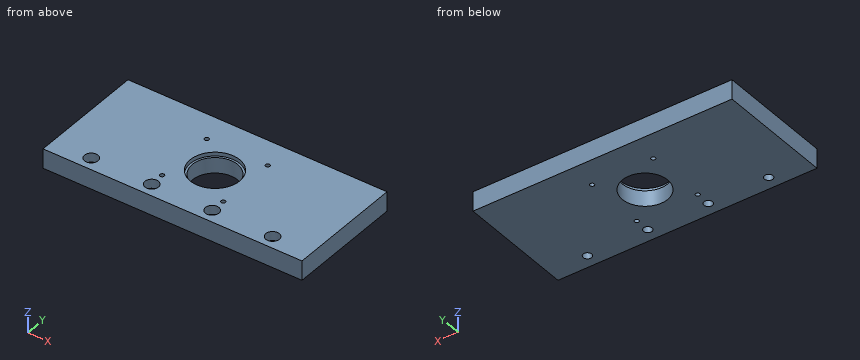
```python
from build123d import *

# Parameters (mm, degrees)
SKETCH_W        = 200
SKETCH_H        = 90
PAD_DEPTH       = 15
SKETCH001_R     = 17.5
SKETCH001_R_2   = 3.25
POCKET_DEPTH    = 15
SKETCH002_R     = 1.65
POCKET001_DEPTH = 15
SKETCH003_R     = 19.1
POCKET002_DEPTH = 3
SKETCH004_R     = 5.2
POCKET003_DEPTH = 7


with BuildPart() as part:
    # Sketch → Pad (new body)
    with BuildSketch(Plane.XY):
        with Locations((100, 45)):
            Rectangle(SKETCH_W, SKETCH_H)
    extrude(amount=PAD_DEPTH)

    # Sketch001 (on Face6 of Pad) → Pocket (cut)
    with BuildSketch(Plane.XY.offset(15)):
        with Locations((100, 45)):
            Circle(SKETCH001_R)
        with Locations((30, 10)):
            Circle(SKETCH001_R_2)
        with Locations((76.67, 10)):
            Circle(SKETCH001_R_2)
        with Locations((123.33, 10)):
            Circle(SKETCH001_R_2)
        with Locations((170, 10)):
            Circle(SKETCH001_R_2)
    extrude(amount=-POCKET_DEPTH, mode=Mode.SUBTRACT)

    # Sketch002 (on Face5 of Pocket) → Pocket001 (cut)
    with BuildSketch(Plane.XY.offset(15)):
        with Locations((76.43, 68.57)):
            Circle(SKETCH002_R)
        with Locations((123.57, 68.57)):
            Circle(SKETCH002_R)
        with Locations((76.43, 21.43)):
            Circle(SKETCH002_R)
        with Locations((123.57, 21.43)):
            Circle(SKETCH002_R)
    extrude(amount=-POCKET001_DEPTH, mode=Mode.SUBTRACT)

    # Sketch003 (on Face5 of Pocket001) → Pocket002 (cut)
    with BuildSketch(Plane.XY.offset(15)):
        with Locations((100, 45)):
            Circle(SKETCH003_R)
    extrude(amount=-POCKET002_DEPTH, mode=Mode.SUBTRACT)

    # Sketch004 (on Face5 of Pocket002) → Pocket003 (cut)
    with BuildSketch(Plane.XY.offset(15)):
        with Locations((30, 10)):
            Circle(SKETCH004_R)
        with Locations((76.67, 10)):
            Circle(SKETCH004_R)
        with Locations((123.33, 10)):
            Circle(SKETCH004_R)
        with Locations((170, 10)):
            Circle(SKETCH004_R)
    extrude(amount=-POCKET003_DEPTH, mode=Mode.SUBTRACT)


solid = part.part
```
Model file for the job. Use its own axes, mm. Give positions to 0.01 mm unless a question says otherwise; leave off trailing zeros. Loops run counter-clockwise (first coordinate to the right, second up) from the corner with the lowest first, then second, coordinate; pieces in that order, holes last. Notation, with made-up numbers: (-5, 60) - (44, 60) arc R21 ccw to (44, 78) - close; hole circle Ø3 at (19.5, 86.25). An arc over 180 degrees is marked (long way). One line per item, written item: value. Start each with the question number.
1. Probe L1, parallel to Y at x = 76.43, z = 5; L2, parallel to Y at x = 100, z = 13.7; L3, parallel to X at y = 46, z = 6. List the from-to ranges inside material, lowest first. Write a range as from..to.
2. Slice it at C-C (x = 170). List the corners of the cut face in (y, z).
3. Slice it at A-A (y = 45). List the corners of the cut face in (x, z).
4. Pin check, flat tips, straight feed: pin 1 (13.5 mm diameter, centred on x = 123.33, y = 10, fed in from +Z); pin 2 (2 mm diameter, centred on x = 115.5, y = 49, fed in from +Z); pin 3 (8.5 mm diameter, centred on x = 123.33, y = 10, fed in from +Z). Stop position of each tip, or through.
5. Slice it at B-B (z = 3.75). Give the number of separate pieces and of enclosed holes in the cut face, plus the area to 3 significant figures.
Solution:
1. L1: y = 0..6.76, 13.24..19.78, 23.08..66.92, 70.22..90
1. L2: y = 0..25.9, 64.1..90
1. L3: x = 0..82.53, 117.47..200
2. outline: (0, 0) - (6.75, 0) - (6.75, 8) - (4.8, 8) - (4.8, 15) - (0, 15) - close; (13.25, 0) - (90, 0) - (90, 15) - (15.2, 15) - (15.2, 8) - (13.25, 8) - close
3. outline: (0, 0) - (82.5, 0) - (82.5, 12) - (80.9, 12) - (80.9, 15) - (0, 15) - close; (117.5, 0) - (200, 0) - (200, 15) - (119.1, 15) - (119.1, 12) - (117.5, 12) - close
4. pin 1: stops at z = 15
4. pin 2: passes through
4. pin 3: stops at z = 8
5. separate pieces: 1
5. enclosed holes: 9
5. area: 16,900 mm^2
